CAD build for the part. Positions are in the model's coordinates, mm. A direction names the side the tool comes from. Coordinates: 2 decimals unless noted, no trailing zeros. Order: outer loops, then holes, each group sorted by start corner. A loop starts at its lowest first (then second) coordinate and runs counter-clockwise, first axis right, second up. Notation, with made-up numbers: (33.5, -13.75) -> (71.5, -13.75) arc R16 ccw to (71.5, -1.75) -> close; hole circle Ø6 at (-4, 21.25). An arc over 180 degrees is marked (long way). Use one line per item in the form item = value. Start each with the question number.
from build123d import *

# Parameters (mm, degrees)
LINEAR_AUSTRAGEN1_DEPTH = 5
SKIZZE2_W               = 6
SKIZZE2_H               = 4
LINEAR_AUSTRAGEN2_DEPTH = 10


with BuildPart() as part:
    # Skizze1 → Linear austragen1 (new body, symmetric)
    with BuildSketch(Plane(origin=(0, 0, 0), x_dir=(0, 0, -1), z_dir=(1, 0, 0))):
        Polygon((0, 0), (1, 0), (1, 5), (-1, 5), (-1, -6), (0, -6), align=None)
    extrude(amount=LINEAR_AUSTRAGEN1_DEPTH, both=True)

    # Skizze2 → Linear austragen2 (cut)
    with BuildSketch(Plane.XY.offset(1)):
        with Locations((0, -2)):
            Rectangle(SKIZZE2_W, SKIZZE2_H)
    extrude(amount=-LINEAR_AUSTRAGEN2_DEPTH, mode=Mode.SUBTRACT)


solid = part.part
1) Probe L1, parallel to X at y = -0.25, z = 0.4; L2, parallel to Y at x = -2, z = 0.6; L3, parallel to Y at x = -4, z = -0.85. List the from-to ranges inside material, lowest first.
2) Drop a flat-ended pin along its axis: P1, Ø1.5, axis at x = -3, y = -2, coming from the -Z side. Give the stop position or say it passes through.
3) Cut at A-A on x = -2.25. Give the cut face in (y, z), then the cut area to 3 significant figures.
4) Two-plate mould, pull along X, no slides. Class faces 3 (the face through (0.1, -4.4, 0)), 4 (the face through (0, 0, 0)), 5 (the face through (-5, 1, 0)): released by +X, released by -X, zero draft, split by the parting line, or undercut.
5) 3-axis set-ups, long thin cutter, end or side, ignore diameter. For faces 1 (the face through (0, 1, 1)), 2 (the face through (3, -2, 0.5)): which of +Z, -Z, +X, -X, +Y, -Y reach the whole face in a straight line?
6) Cut at C-C on x = -3.5. Give the cut face in (y, z).
7) Cut at B-B on z = 0.55. Give the cut face in (x, y).
8) Cut at D-D on y = -5. Give the cut face in (x, z), then the cut area to 3 significant figures.
Values follow:
q1.L1 = -5 to -3, 3 to 5
q1.L2 = -6 to -4, 0 to 5
q1.L3 = 0 to 5
q2.P1 = 0
q3.outline = (-6, 0) -> (-4, 0) -> (-4, 1) -> (-6, 1) -> close; (0, -1) -> (5, -1) -> (5, 1) -> (0, 1) -> close
q3.area = 12.0 mm^2
q4.face_3 = zero draft
q4.face_4 = undercut
q4.face_5 = released by -X
q5.face_1 = +Z, +X, -X, +Y, -Y
q5.face_2 = +Z, -Z
q6.outline = (-6, 0) -> (0, 0) -> (0, -1) -> (5, -1) -> (5, 1) -> (-6, 1) -> close
q7.outline = (-5, -6) -> (5, -6) -> (5, 5) -> (-5, 5) -> close; hole (-3, -4) -> (3, -4) -> (3, 0) -> (-3, 0) -> close
q8.outline = (-5, 0) -> (5, 0) -> (5, 1) -> (-5, 1) -> close
q8.area = 10.0 mm^2
